Source: three-view drawing plus pictorial views. Frame: mm from the lowest corner of the part. Coordinates: 2 decimals unless noted, no trailing zeros. Write each loop counter-clockwise with the first axis right and the second up, starting at its lowest first coordinate (ties: lowest second). Pieces come first, ordered by that corner, then holes. Notation, with made-up numbers: (58.5, 73) -> (71.5, 73) arc R9 ccw to (71.5, 79) -> close; hole circle Ø8 at (23, -23). An arc over 180 degrees is marked (long way). One line per item, written item: value.
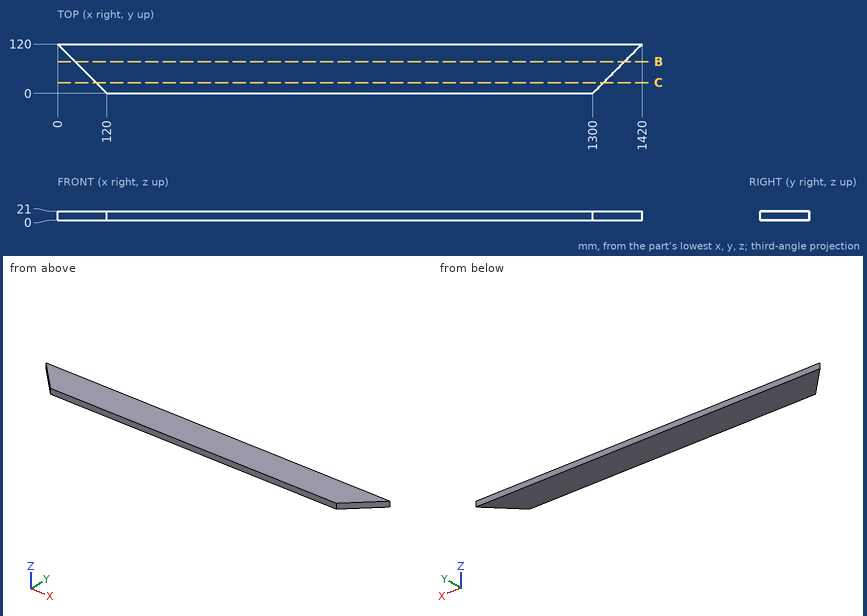
(1) First-contact query: pin 1 (2 mm diameter, centred on y = 45.5, z = 8, fed in from -X); pin 2 (5 mm diameter, centred on x = 520, y = 100, fed in from -Z); pin 3 (10 mm diameter, centred on y = 86, z = 12.5, fed in from +X). Flat tips, straight axial feed; report the tip coordinate or a pass-through.
Responses:
pin 1: stops at x = 73.5
pin 2: stops at z = 0
pin 3: stops at x = 1391
(2) Section C-C (y = 26). Return the cut outline in (x, z).
Responses:
outline: (94, 0) -> (1326, 0) -> (1326, 21) -> (94, 21) -> close
(3) Section B-B (y = 77). Return the cut outline in (x, z), then the cut area to 3 significant figures.
Responses:
outline: (43, 0) -> (1377, 0) -> (1377, 21) -> (43, 21) -> close
area: 28,000 mm2
(4) Line query: line 1 (X direction, y = 69, z = 1.75); line 2 (X direction, y = 111, z = 6.5); line 3 (Y direction, x = 95.5, z = 1.5). Output: solid intervals per line, ascending. Write a range as [from, to].
Responses:
line 1: x = [51, 1369]
line 2: x = [9, 1411]
line 3: y = [24.5, 120]
